Geometry check sheet. Reference: drawing and pictorial views, mm from the part's lowest x, y, z. Give positions to 0.01 mm unless a question says otherwise; leave off trailing zeros. Order: outer loops, then holes, each group sorted by start corner. A loop starts at its lowest first (then second) coordinate and runs counter-clockwise, first axis right, second up. Notation, with made-up numbers: (86.5, -14.75) - (140.5, -14.75) arc R26 cw to (140.5, -0.75) - close; hole circle Ø2 at (62.5, -9.75). An arc over 180 degrees is marked (long way). Answer in a Markdown table with one row per item.
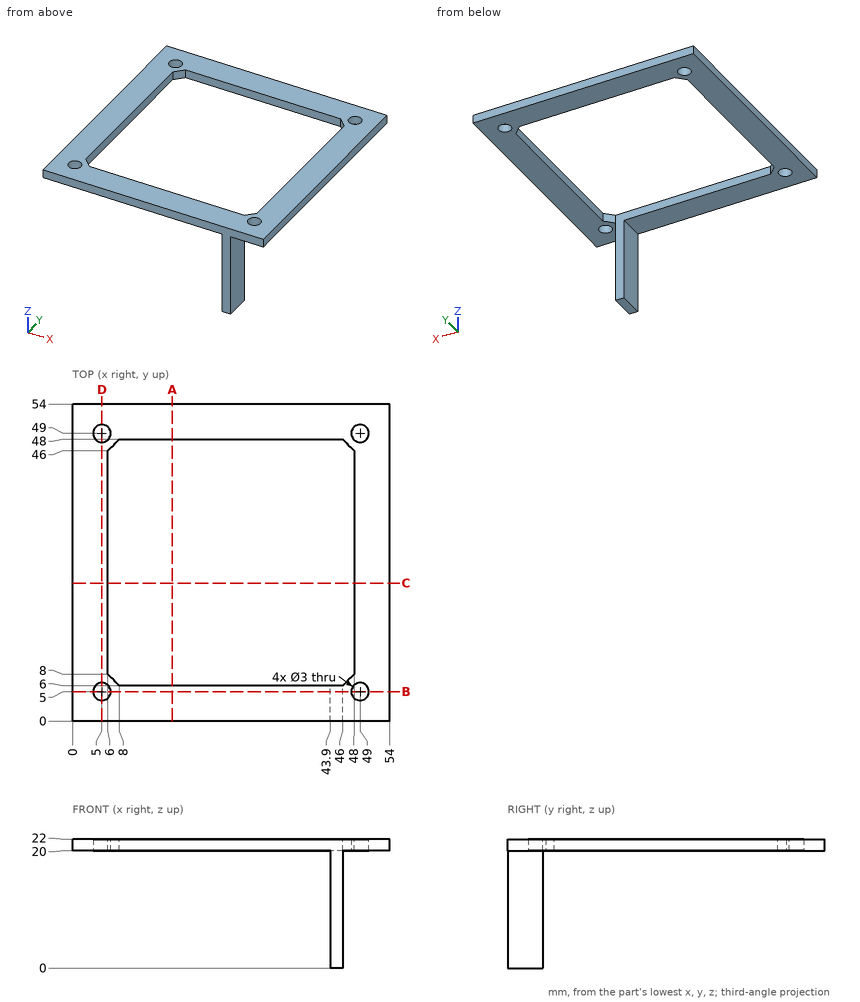
(1) Cross-section at D-D, the plane x = 5. Record the cut outline in (y, z).
Geometry says:
| item | result |
|---|---|
| outline | (0, 20) - (3.5, 20) - (3.5, 22) - (0, 22) - close; (6.5, 20) - (47.5, 20) - (47.5, 22) - (6.5, 22) - close; (50.5, 20) - (54, 20) - (54, 22) - (50.5, 22) - close |
(2) Gauge pin test, flat ends, axial feed: P1, Ø12, axis at x = 16.5, y = 6.5, coming from the +Z side; P2, Ø5, axis at y = 2.5, z = 9.5, coming from the -X side; P3, Ø4, axis at x = 49, y = 49, coming from the -Z side; P4, Ø6, axis at y = 6.5, z = 12, coming from the +X side. Record the tip position at first contact, or that the pin passes through.
Geometry says:
| item | result |
|---|---|
| P1 | z = 22 |
| P2 | x = 43.9 |
| P3 | z = 20 |
| P4 | x = 46 |
(3) Cross-section at A-A, the plane x = 17. Record the cut outline in (y, z).
Geometry says:
| item | result |
|---|---|
| outline | (0, 20) - (6, 20) - (6, 22) - (0, 22) - close; (48, 20) - (54, 20) - (54, 22) - (48, 22) - close |
(4) Thickness scan on L1, parallel to Y at x = 5, z = 21.5; L2, parallel to X at y = 4, z = 14.25; L3, parallel to Z at x = 50, y = 8. Record the ranges inside material, lowest first.
Geometry says:
| item | result |
|---|---|
| L1 | 0 to 3.5, 6.5 to 47.5, 50.5 to 54 |
| L2 | 43.9 to 46 |
| L3 | 20 to 22 |
(5) Cross-section at B-B, the plane y = 5. Record the cut outline in (x, z), then the cut area to 3 significant figures.
Geometry says:
| item | result |
|---|---|
| outline | (0, 20) - (3.5, 20) - (3.5, 22) - (0, 22) - close; (6.5, 20) - (43.9, 20) - (43.9, 0) - (46, 0) - (46, 20) - (47.5, 20) - (47.5, 22) - (6.5, 22) - close; (50.5, 20) - (54, 20) - (54, 22) - (50.5, 22) - close |
| area | 138 mm² |
